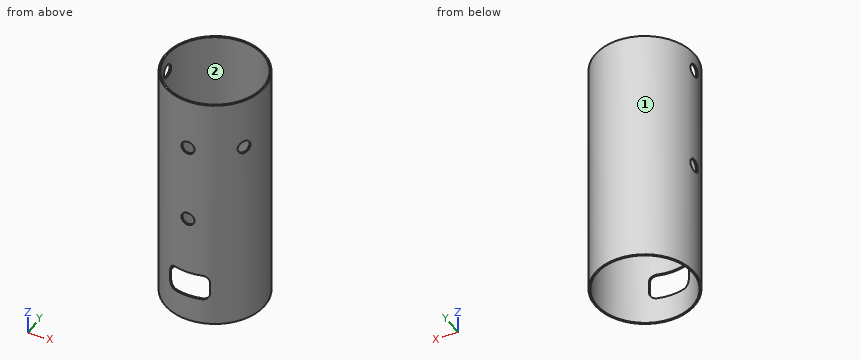
```python
from build123d import *

# Parameters (mm, degrees)
F0_R          = 37.5
F0_R_2        = 36.25
F1_DEPTH      = 184
F2_R          = 5
F3_DEPTH      = 50
F4_R          = 5
F5_DEPTH      = 70
F5_DEPTH_BACK = 25
F7_DEPTH      = 70
F8_R          = 5
F9_DEPTH      = 60
F12_R         = 5
F13_DEPTH     = 100


with BuildPart() as f1:
    # F0 (on Top) → F1 (new body)
    with BuildSketch(Plane.XY):
        Circle(F0_R)
        Circle(F0_R_2, mode=Mode.SUBTRACT)
    extrude(amount=F1_DEPTH)

    # F2 (on Right) → F3 (cut)
    with BuildSketch(Plane.YZ):
        with Locations((0, 170)):
            Circle(F2_R)
    extrude(amount=-F3_DEPTH, mode=Mode.SUBTRACT)

    # F4 (on Front) → F5 (cut, two sides)
    with BuildSketch(Plane.XZ) as f5_sk:
        with Locations((0, 85)):
            Circle(F4_R)
        with Locations((0, 145)):
            Circle(F4_R)
    extrude(amount=F5_DEPTH, mode=Mode.SUBTRACT)
    extrude(f5_sk.sketch, amount=-F5_DEPTH_BACK, mode=Mode.SUBTRACT)

    # F6 (on Front) → F7 (cut)
    with BuildSketch(Plane.XZ):
        with BuildLine():
            Line((-10, 20), (10, 20))
            ThreePointArc((10, 20), (13.535534, 21.464466), (15, 25))
            Line((15, 25), (15, 35))
            ThreePointArc((15, 35), (13.535534, 38.535534), (10, 40))
            Line((10, 40), (-10, 40))
            ThreePointArc((-10, 40), (-13.535534, 38.535534), (-15, 35))
            Line((-15, 35), (-15, 25))
            ThreePointArc((-15, 25), (-13.535534, 21.464466), (-10, 20))
        make_face()
    extrude(amount=F7_DEPTH, mode=Mode.SUBTRACT)

    # F8 (on Right) → F9 (cut)
    with BuildSketch(Plane.YZ):
        with Locations((0, 90)):
            Circle(F8_R)
    extrude(amount=-F9_DEPTH, mode=Mode.SUBTRACT)

    # F12 (on face) → F13 (cut)
    with BuildSketch(Plane(origin=(0, 0, 0), x_dir=(0.5, 0.866025, 0), z_dir=(0.866025, -0.5, 0))):
        with Locations((0, 145)):
            Circle(F12_R)
    extrude(amount=F13_DEPTH, mode=Mode.SUBTRACT)


solid = f1.part
```
Can you work these out from the model? Positions are in its coordinate system, mm. Face numbers are marked on the shaded views. Round coordinates to 2 decimals unless told otherwise and drop trailing zeros. Loops run counter-clockwise (first coordinate to the right, second up) from the corner with the lowest first, then second, coordinate; pieces in that order, holes last.
Item 1: Please list where these lines run through material, in increasing order: L1, parallel to Z at x = 0, y = -37.1; L2, parallel to X at y = 0, z = 133.5; L3, parallel to X at y = 7.5, z = 83.5.
Item 2: If we mould it in two halves opening along X, with no side actions, what happens to the marked faces 1 and 2? For each: +X half, -X half, draft (parallel to the pull), parting line (faces both ways), or undercut.
Item 3: Will these pins go through, and if not, where does the flat tip stop? pin 1 Ø4 at (y, z) = (12, 160.5) entering from -X; pin 2 Ø10 at (x, z) = (7.5, 91.5) entering from -Y; pin 3 Ø3 at (y, z) = (-22.5, 24) entering from +X; pin 4 Ø10 at (x, y) = (-20, 21) entering from -Z.
Item 4: Suppose I cut it at A-A, the plane x = 0. Write out the boundary of the cut face in (y, z), then the cut area to 3 significant figures.
Item 5: Suppose I cut it at B-B, the plane y = 0. Write out the boundary of the cut face in (x, z), then the cut area to 3 significant figures.
Item 6: Suppose I cut it at C-C, the plane x = -20. Write out the boundary of the cut face in (y, z).
Item 7: Suppose I cut it at D-D, the plane z = 145. Write out the boundary of the cut face in (x, y), then the cut area to 3 significant figures.
Reported:
1. L1: z = 0 to 20, 40 to 80, 90 to 140, 150 to 184
1. L2: x = -37.5 to -36.25, 36.25 to 37.5
1. L3: x = -36.74 to -35.47, 35.47 to 36.74
2. face 1: parting line
2. face 2: undercut
3. pin 1: stops at x = -36.14
3. pin 2: stops at y = -37.42
3. pin 3: stops at x = 31.07
3. pin 4: passes through
4. outline: (-37.5, 0) - (-36.25, 0) - (-36.25, 20) - (-37.5, 20) - close; (-37.5, 40) - (-36.25, 40) - (-36.25, 80) - (-37.5, 80) - close; (-37.5, 90) - (-36.25, 90) - (-36.25, 140) - (-37.5, 140) - close; (-37.5, 150) - (-36.25, 150) - (-36.25, 184) - (-37.5, 184) - close; (36.25, 0) - (37.5, 0) - (37.5, 184) - (36.25, 184) - close
4. area: 410 mm2
5. outline: (-37.5, 0) - (-36.25, 0) - (-36.25, 85) - (-37.5, 85) - close; (-37.5, 95) - (-36.25, 95) - (-36.25, 165) - (-37.5, 165) - close; (-37.5, 175) - (-36.25, 175) - (-36.25, 184) - (-37.5, 184) - close; (36.25, 0) - (37.5, 0) - (37.5, 184) - (36.25, 184) - close
5. area: 435 mm2
6. outline: (-31.72, 0) - (-30.23, 0) - (-30.23, 184) - (-31.72, 184) - close; (30.23, 0) - (31.72, 0) - (31.72, 184) - (30.23, 184) - close
7. outline: (-5, -37.17) - (-5, -35.9) arc R36.25 cw (long way) to (33.59, -13.62) - (34.69, -14.25) arc R37.5 ccw (long way) to start; (5, -37.17) arc R37.5 ccw to (29.69, -22.91) - (28.59, -22.28) arc R36.25 cw to (5, -35.9) - close
7. area: 265 mm2
